Check sheet for the modelled part. Datum: model origin and axes. Units: mm. Face numbers are marked on the shaded views. A direction names the side the tool comes from. Give positions to 0.01 mm unless a question says otherwise; leave off trailing zeros. Order: outer loops, then holes, each group sorted by start corner. A loop starts at its lowest first (then second) coordinate and runs counter-clockwise, first axis right, second up.
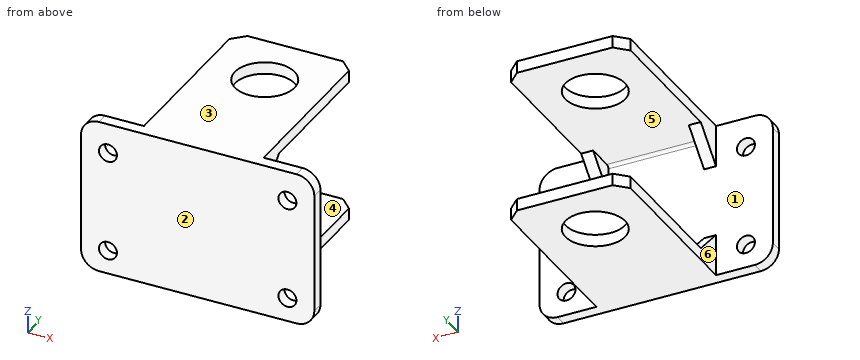
```python
from build123d import *

# Parameters (mm, degrees)
SKETCH1_W            = 20
SKETCH1_H            = 26
BOSS_EXTRUDE1_DEPTH  = 2
SKETCH2_W            = 20
SKETCH2_H            = 2
BOSS_EXTRUDE2_DEPTH  = 30
SKETCH3_R            = 5
CUT_EXTRUDE1_DEPTH   = 43.426406871
SKETCH4_W            = 39
SKETCH4_H            = 26
BOSS_EXTRUDE3_DEPTH  = 2
SKETCH5_R            = 1.5
CUT_EXTRUDE2_DEPTH   = 39.069016273
FILLET1_R            = 3
CHAMFER1_SIZE        = 2
RIB3_START           = -2
RIB3_DEPTH           = 2
MIRROR2_START        = -2
MIRROR2_COPY_1_DEPTH = 2
FILLET2_R            = 0.5


# Read off the part's stored shape, not the designer's step: Rib3
with BuildPart() as part:
    # Sketch1 → Boss-Extrude1 (new body)
    with BuildSketch(Plane(origin=(0, 0, 0), x_dir=(1, 0, 0), z_dir=(0, 1, 0))):
        Rectangle(SKETCH1_W, SKETCH1_H)
    extrude(amount=BOSS_EXTRUDE1_DEPTH)

    # Sketch2 → Boss-Extrude2 (add)
    with BuildSketch(Plane(origin=(0, 2, 0), x_dir=(1, 0, 0), z_dir=(0, 1, 0))):
        with Locations((0, -12)):
            Rectangle(SKETCH2_W, SKETCH2_H)
        with Locations((0, 12)):
            Rectangle(SKETCH2_W, SKETCH2_H)
    extrude(amount=BOSS_EXTRUDE2_DEPTH)

    # Sketch3 → Cut-Extrude1 (cut, through all)
    with BuildSketch(Plane.XY.offset(13)):
        with Locations((0, 22)):
            Circle(SKETCH3_R)
    extrude(amount=-CUT_EXTRUDE1_DEPTH, mode=Mode.SUBTRACT)

    # Sketch4 → Boss-Extrude3 (add)
    with BuildSketch(Plane(origin=(0, 2, 0), x_dir=(1, 0, 0), z_dir=(0, 1, 0))):
        Rectangle(SKETCH4_W, SKETCH4_H)
    extrude(amount=-BOSS_EXTRUDE3_DEPTH)

    # Sketch5 → Cut-Extrude2 (cut, through all)
    with BuildSketch(Plane(origin=(0, 2, 0), x_dir=(1, 0, 0), z_dir=(0, 1, 0))):
        with Locations(Location((-15, 9.01, 0), (0, 0, 270))):
            Circle(SKETCH5_R)
        with Locations(Location((-15, -7.99, 0), (0, 0, 270))):
            Circle(SKETCH5_R)
        with Locations(Location((15, -7.99, 0), (0, 0, 270))):
            Circle(SKETCH5_R)
        with Locations(Location((15, 9.01, 0), (0, 0, 270))):
            Circle(SKETCH5_R)
    extrude(amount=-CUT_EXTRUDE2_DEPTH, mode=Mode.SUBTRACT)

    # Fillet1
    fillet1_edges = [part.edges().sort_by_distance(p)[0] for p in [
        (-19.5, 1, -13),
        (19.5, 1, 13),
        (-19.5, 1, 13),
        (19.5, 1, -13),
    ]]
    fillet(fillet1_edges, radius=FILLET1_R)

    # Chamfer1
    chamfer1_edges = [part.edges().sort_by_distance(p)[0] for p in [
        (10, 32, 12),
        (-10, 32, 12),
        (-10, 32, -12),
        (10, 32, -12),
    ]]
    chamfer(chamfer1_edges, length=CHAMFER1_SIZE)

    # Rib3 outline → Rib3 (add)
    with BuildSketch(Plane(origin=(10, 0, 0), x_dir=(0, 0, -1), z_dir=(1, 0, 0)).offset(RIB3_START)):
        Polygon((11, 2), (11, 7), (6, 2), align=None)
    rib3 = extrude(amount=RIB3_DEPTH)

    # Mirror1: Rib3 across plane
    add(rib3.mirror(Plane.XY))

    # Mirror2: Rib3 across plane
    add(rib3.mirror(Plane(origin=(0, 0, 0), x_dir=(0, 0, 1), z_dir=(1, 0, 0))))

    # Mirror2 copy 1 sketch → Mirror2 copy 1 (add)
    with BuildSketch(Plane.ZY.offset(10).offset(MIRROR2_START)):
        Polygon((11, 2), (11, 7), (6, 2), align=None)
    extrude(amount=MIRROR2_COPY_1_DEPTH)

    # Fillet2
    fillet2_edges = [part.edges().sort_by_distance(p)[0] for p in [
        (0, 2, 11),
        (0, 2, -11),
    ]]
    fillet(fillet2_edges, radius=FILLET2_R)


solid = part.part
```
(1) Cross-section at B-B on x = 15. Enter the section's corners in (y, z), then the cut area to 3 significant figures.
Response values:
outline: (0, -13) - (2, -13) - (2, -10.51) - (0, -10.51) - close; (0, -7.51) - (2, -7.51) - (2, 6.49) - (0, 6.49) - close; (0, 9.49) - (2, 9.49) - (2, 13) - (0, 13) - close
area: 40.0 mm2
(2) Material ranges on L1, parallel to X at y = 0.55, z = -9.01; L2, parallel to Y at x = 0, z = 12.6; L3, parallel to Z at x = -7, y = 26, recorded low to high.
Response values:
L1: x = -19.5 to -16.5, -13.5 to 13.5, 16.5 to 19.5
L2: y = 0 to 17, 27 to 32
L3: z = -13 to -11, 11 to 13
(3) Cross-section at A-A on y = 22. Enter the section's corners in (x, z), then the cut area to 3 significant figures.
Response values:
outline: (-10, -13) - (-5, -13) - (-5, -11) - (-10, -11) - close; (-10, 11) - (-5, 11) - (-5, 13) - (-10, 13) - close; (5, -13) - (10, -13) - (10, -11) - (5, -11) - close; (5, 11) - (10, 11) - (10, 13) - (5, 13) - close
area: 40.0 mm2
(4) Cross-section at C-C on z = 7.99. Enter the section's corners in (x, y).
Response values:
outline: (-19.5, 0) - (-16.5, 0) - (-16.5, 2) - (-19.5, 2) - close; (-13.5, 0) - (13.5, 0) - (13.5, 2) - (10, 2) - (10, 3.99) - (8, 3.99) - (8, 2) - (-8, 2) - (-8, 3.99) - (-10, 3.99) - (-10, 2) - (-13.5, 2) - close; (16.5, 0) - (19.5, 0) - (19.5, 2) - (16.5, 2) - close
(5) Release check for a two-part mould opening along Z. For the marked faces 3, 4, 5 and 6 record: released by +Z, released by -Z, zero draft, split by the parting line, or undercut.
Response values:
face 3: released by +Z
face 4: undercut
face 5: undercut
face 6: zero draft
(6) Set-up check for the marked faces 1 and 2: record each of +Z, -Z, +X, -X, +Y, -Y from which the full face is reachable in a straight line by a thin tool's end or side.
Response values:
face 1: +Y
face 2: +Z, -Z, +X, -X, -Y
(7) Gauge pin test, flat ends, axial feed: pin 1 Ø3.5 at (y, z) = (12, 8) entering from +X; pin 2 Ø1 at (x, z) = (14, 9) entering from +Y; pin 3 Ø6 at (y, z) = (12, 10) entering from +X; pin 4 Ø2.5 at (y, z) = (3.5, -9.5) entering from -X. Record the tip position at first contact, or that the pin passes through.
Response values:
pin 1: passes through
pin 2: stops at y = 2
pin 3: stops at x = 10
pin 4: stops at x = -10
(8) Cross-section at D-D on y = 11.5. Enter the section's corners in (x, z).
Response values:
outline: (-10, -13) - (10, -13) - (10, -11) - (-10, -11) - close; (-10, 11) - (10, 11) - (10, 13) - (-10, 13) - close
